Check sheet for the modelled part. Datum: model origin and axes. Units: mm. Face numbers are marked on the shaded views. A direction names the side the tool comes from. Give positions to 0.01 mm unless a question says otherwise; leave off trailing zeros. Write each loop counter-clockwise with the first axis right and the second up, starting at its lowest first coordinate (ties: lowest second). Pieces come first, ordered by that corner, then holes. Notation, with made-up numbers: M -4.75,12.5 L 21.25,12.5 A19 ccw 21.25,44.5 Z; hole C -38,9.25 d4. An arc over 180 degrees is marked long. Use CSV: the item, a comma, the result in double quotes. Start each with the question number.
1. Cross-section at B-B, the plane x = 1. Enter the section's corners in (y, z).
2. Depth check by flat-ended pin: P1, Ø8, axis at x = -6.5, y = -8.5, coming from the +Z side; P2, Ø7.5, axis at x = 2, z = 39.5, coming from the +Y side; P3, Ø6, axis at x = 17, y = 9.5, coming from the +Z side. Enter the tip coordinate at first touch or a pass-through.
3. Scan lines: line 1 (Y direction, x = -23, z = 39); line 2 (Z direction, x = 18, y = 10); line 3 (Y direction, x = 24, z = 28.5). Record each from-to range of solid material in increasing order.
4. Cross-section at A-A, the plane z = 37. Enter the section's corners in (x, y).
5. Cross-section at D-D, the plane z = 22. Enter the section's corners in (x, y), and give its area (3 significant figures).
6. Mould release check, pull along Y, two halves, no side actions. Record for the marked faces 4, 5 and 6: +Y half, -Y half, draft (parallel to the pull), parting line (faces both ways), or undercut.
7. Cross-section at C-C, the plane y = 15. Enter the section's corners in (x, z).
8. Access from +Z, -Z, +X, -X, +Y, -Y to the whole of each face (thin tool, end or side, straight path). Record for the marked faces 1, 2 and 3.
from build123d import *

# Parameters (mm, degrees)
F0_W     = 65
F0_H     = 4.5996872587
F0_H_2   = 9.9056614563
F1_DEPTH = 10
F2_DEPTH = 50
F3_DEPTH = 35
F4_R     = 2


with BuildPart() as f1:
    # F0 (on Top) → F1 (new body)
    with BuildSketch(Plane.XY):
        with BuildLine():
            ThreePointArc((32.5, 35), (31.0355339059, 38.5355339059), (27.5, 40))
            Line((27.5, 40), (-27.5, 40))
            ThreePointArc((-27.5, 40), (-31.0355339059, 38.5355339059), (-32.5, 35))
            Line((-32.5, 35), (-32.5, 1.505348715))
            Line((-32.5, 1.505348715), (32.5, 1.505348715))
            Line((32.5, 1.505348715), (32.5, 35))
        make_face()
        with Locations((0, -0.7944949144)):
            Rectangle(F0_W, F0_H)
        with Locations((0, -8.0471692719)):
            Rectangle(F0_W, F0_H_2)
        with BuildLine():
            Line((32.5, -35), (32.5, -13))
            Line((32.5, -13), (-32.5, -13))
            Line((-32.5, -13), (-32.5, -35))
            ThreePointArc((-32.5, -35), (-31.0355339059, -38.5355339059), (-27.5, -40))
            Line((-27.5, -40), (27.5, -40))
            ThreePointArc((27.5, -40), (31.0355339059, -38.5355339059), (32.5, -35))
        make_face()
    extrude(amount=F1_DEPTH)

    # F0 (on Top) → F2 (join)
    with BuildSketch(Plane.XY):
        with Locations((0, -0.7944949144)):
            Rectangle(F0_W, F0_H)
        with BuildLine():
            Line((32.5, -35), (32.5, -13))
            Line((32.5, -13), (-32.5, -13))
            Line((-32.5, -13), (-32.5, -35))
            ThreePointArc((-32.5, -35), (-31.0355339059, -38.5355339059), (-27.5, -40))
            Line((-27.5, -40), (27.5, -40))
            ThreePointArc((27.5, -40), (31.0355339059, -38.5355339059), (32.5, -35))
        make_face()
    extrude(amount=F2_DEPTH)

    # F0 (on Top) → F3 (join)
    with BuildSketch(Plane.XY):
        with Locations((0, -8.0471692719)):
            Rectangle(F0_W, F0_H_2)
    extrude(amount=F3_DEPTH)

    # F4
    f4_edges = [f1.edges().sort_by_distance(p)[0] for p in [
        (-32.5, -24, 50),
        (32.5, -24, 50),
    ]]
    fillet(f4_edges, radius=F4_R)


solid = f1.part
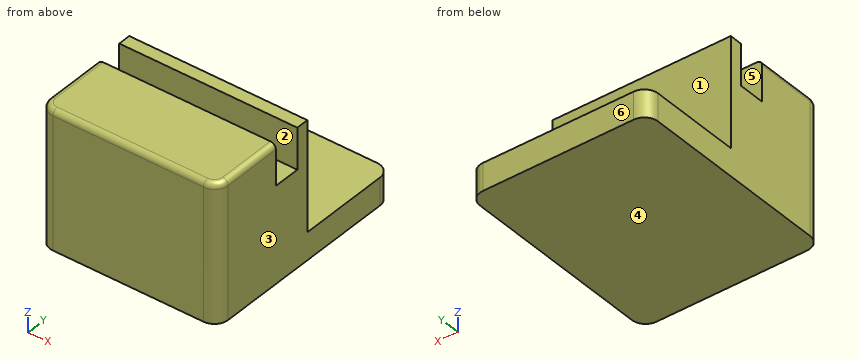
Worked answers:
1,outline,"M -40,0 L 40,0 L 40,10 L 1.51,10 L 1.51,50 L -3.09,50 L -3.09,35 L -13,35 L -13,50 L -38,50 A2 ccw -40,48 Z"
2,P1,"stops at z = 35"
2,P2,"stops at y = 1.51"
2,P3,"stops at z = 10"
3,line 1,"y = -40 to -13, -3.09 to 1.51"
3,line 2,"z = 0 to 10"
3,line 3,"y = -40 to 1.51"
4,outline,"M -32.5,-35 A5 ccw -27.5,-40 L 27.5,-40 A5 ccw 32.5,-35 L 32.5,-13 L -32.5,-13 Z; M -32.5,-3.09 L 32.5,-3.09 L 32.5,1.51 L -32.5,1.51 Z"
5,outline,"M -32.5,-35 A5 ccw -27.5,-40 L 27.5,-40 A5 ccw 32.5,-35 L 32.5,1.51 L -32.5,1.51 Z"
5,area,"2,690 mm^2"
6,face 4,"draft"
6,face 5,"undercut"
6,face 6,"+Y half"
7,outline,"M -32.5,0 L 32.5,0 L 32.5,10 L -32.5,10 Z"
8,face 1,"+Z, +X, -X, +Y"
8,face 2,"+Z, +X, -X"
8,face 3,"+Z, -Z, +X, +Y, -Y"
